Check sheet for the drawn part. Datum: minimum x, y, z corner. Units: mm. Coordinates: 2 decimals unless noted, no trailing zeros. Write each loop counter-clockwise with the first axis right and the second up, starting at its lowest first coordinate (ties: lowest second). Pieces come first, ordered by that corner, then holes. Notation, with made-up numbers: M 13,-27 L 59,-27 A13 cw 59,-13 Z; hole C 54.5,8 d1. An arc over 180 degrees is marked long. Answer as CSV lines item,"result".
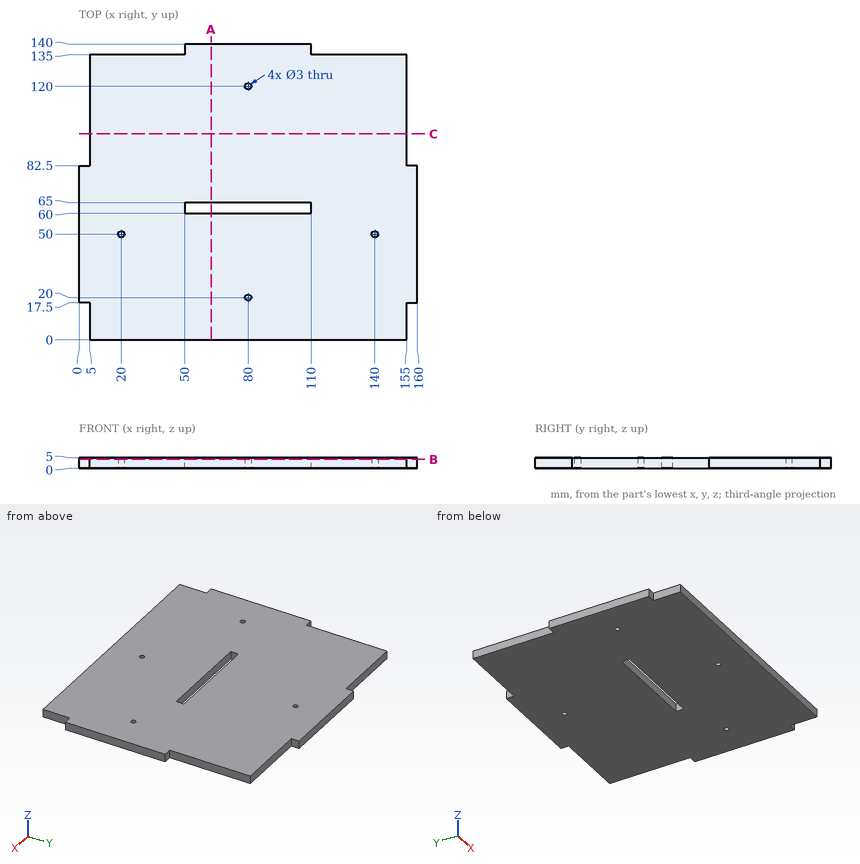
1) Section check A-A, the plane x = 62.5. Record the boundary of the cut face in (y, z), plus the area to 3 significant figures.
Answer key:
outline,"M 0,0 L 60,0 L 60,5 L 0,5 Z; M 65,0 L 140,0 L 140,5 L 65,5 Z"
area,"675 mm2"
2) Section check C-C, the plane y = 97.5. Record the boundary of the cut face in (x, z).
Answer key:
outline,"M 5,0 L 155,0 L 155,5 L 5,5 Z"
3) Section check B-B, the plane z = 4.25. Record the boundary of the cut face in (x, y), plus the area to 3 significant figures.
Answer key:
outline,"M 0,17.5 L 5,17.5 L 5,0 L 155,0 L 155,17.5 L 160,17.5 L 160,82.5 L 155,82.5 L 155,135 L 110,135 L 110,140 L 50,140 L 50,135 L 5,135 L 5,82.5 L 0,82.5 Z; hole C 20,50 d3; hole M 50,60 L 110,60 L 110,65 L 50,65 Z; hole C 80,20 d3; hole C 80,120 d3; hole C 140,50 d3"
area,"20,900 mm2"
4) Thickness scan on line 1 along Y through (x, z) = (80, 1.85); line 2 along X through (y, z) = (50, 3.8); line 3 along Y through (x, z) = (140, 2.45). Record the ranges inside material, lowest first.
Answer key:
line 1,"y = 0 to 18.5, 21.5 to 60, 65 to 118.5, 121.5 to 140"
line 2,"x = 0 to 18.5, 21.5 to 138.5, 141.5 to 160"
line 3,"y = 0 to 48.5, 51.5 to 135"
5) Depth check by flat-ended pin: P1, Ø1.5, axis at y = 107, z = 3.5, coming from the +X side; P2, Ø1.5, axis at y = 10.5, z = 3, coming from the -X side; P3, Ø2.5, axis at x = 80, y = 120, coming from the -Z side; P4, Ø2.5, axis at x = 2.5, z = 3, coming from the -Y side. Enter the tip coordinate at first touch or a pass-through.
Answer key:
P1,"stops at x = 155"
P2,"stops at x = 5"
P3,"passes through"
P4,"stops at y = 17.5"
